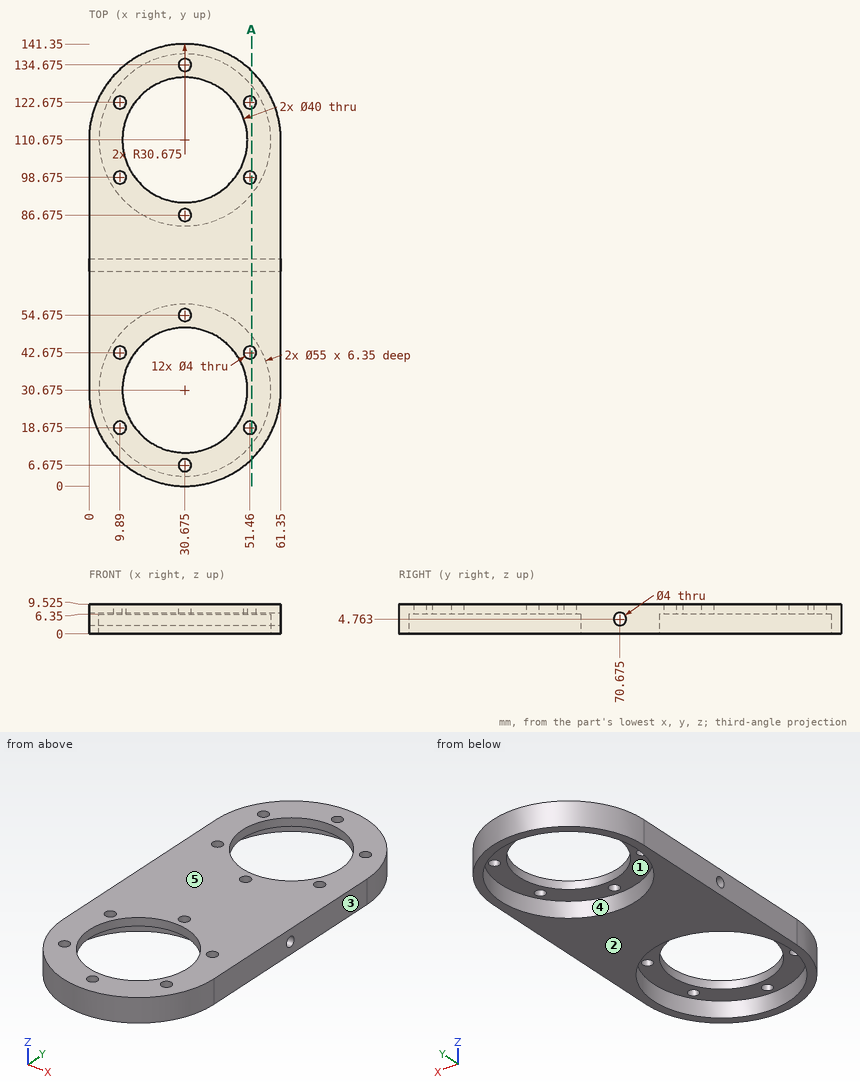
Design review of the part shown in the three views and the two pictorial views. Dimensions are in mm from the part's minimum x, y and z. A direction names the side the tool comes from. Round coordinates to 2 decimals unless told otherwise and drop trailing zeros. Answer as a JSON object with one key per item and string values.
Item 1: Wall thickness on L1, parallel to Z at x = 33, y = 70.5 (1 decimal); L2, parallel to Y at x = 26.5, z = 1 (1 decimal); L3, parallel to Y at x = 24, z = 5.5 (1 decimal): over which ranges is each line inside the solid? List them lowest first. Write a range as from..to.
Answer sheet:
{"L1": "z = 0..2.8, 6.8..9.5", "L2": "y = 0.3..3.5, 57.9..83.5, 137.9..141.1", "L3": "y = 0.7..4, 57.4..68.8, 72.5..84, 137.4..140.6"}
Item 2: We need section A-A on x = 52. State how many separate pieces and enclosed holes the cut face has.
Answer sheet:
{"separate pieces": "5", "enclosed holes": "1"}
Item 3: The part is to be moulded in two halves that separate along X. For the marked faces 3, 4 and 5, say which applies: pulls with the +X half, pulls with the -X half, needs draft (parallel to the pull), parting line crosses it, or undercut.
Answer sheet:
{"face 3": "pulls with the +X half", "face 4": "undercut", "face 5": "needs draft"}
Item 4: Clearance check with flat-ended pins moving along their axes: P1, Ø5, axis at x = 9.89, y = 122.68, coming from the -Z side; P2, Ø2, axis at y = 121.5, z = 4.5, coming from the -X side (1 decimal); P3, Ø1.5, axis at x = 47, z = 7, coming from the +Y side; P4, Ø3.5, axis at x = 9.89, y = 98.68, coming from the -Z side. State where each tip first meets the part, or that it passes through.
Answer sheet:
{"P1": "stops at z = 6.35", "P2": "stops at x = 1.6", "P3": "stops at y = 137.1", "P4": "passes through"}
Item 5: Machinability: for the marked faces 1 and 2, which of the approach directions +Z, -Z, +X, -X, +Y, -Y give a long, thin tool a straight path to every point of the face, cutting with its end or side? Answer none if there is none.
Answer sheet:
{"face 1": "-Z", "face 2": "-Z, +X, -X, +Y, -Y"}
